from build123d import *

# Parameters (mm, degrees)
SKETCH1_W           = 60
SKETCH1_H           = 32
BOSS_EXTRUDE1_DEPTH = 1.2
BOSS_EXTRUDE2_DEPTH = 5.2
SKETCH3_W           = 10
SKETCH3_H           = 32
BOSS_EXTRUDE3_DEPTH = 1.2
SKETCH4_W           = 15
SKETCH4_H           = 10
BOSS_EXTRUDE4_DEPTH = 1.2
FILLET1_R           = 5
CUT_EXTRUDE1_REACH  = 59.861
SKETCH5_R           = 3.1


with BuildPart() as part:
    # Sketch1 → Boss-Extrude1 (new body)
    with BuildSketch(Plane(origin=(0, 0, 0), x_dir=(1, 0, 0), z_dir=(0, 1, 0))):
        Rectangle(SKETCH1_W, SKETCH1_H)
    extrude(amount=BOSS_EXTRUDE1_DEPTH)

    # Sketch2 → Boss-Extrude2 (add)
    with BuildSketch(Plane.XZ):
        Polygon((-30, -17.2), (31.2, -17.2), (31.2, 17.2), (-30, 17.2), (-30, 16), (30, 16), (30, -16), (-30, -16), align=None)
    extrude(amount=-BOSS_EXTRUDE2_DEPTH)

    # Sketch3 → Boss-Extrude3 (add)
    with BuildSketch(Plane.XZ):
        with Locations((-35, 0)):
            Rectangle(SKETCH3_W, SKETCH3_H)
    extrude(amount=-BOSS_EXTRUDE3_DEPTH)

    # Sketch4 → Boss-Extrude4 (add)
    with BuildSketch(Plane.XZ):
        with Locations((-47.5, 0)):
            Rectangle(SKETCH4_W, SKETCH4_H)
    extrude(amount=-BOSS_EXTRUDE4_DEPTH)

    # Fillet1
    fillet1_edges = [part.edges().sort_by_distance(p)[0] for p in [
        (-55, 0.6, 5),
        (-55, 0.6, -5),
    ]]
    fillet(fillet1_edges, radius=FILLET1_R - 0.0001)  # a hair under: the kernel refuses the full size

    # Sketch5 → Cut-Extrude1 (cut, up to next)
    with BuildSketch(Plane.XZ, mode=Mode.PRIVATE) as cut_extrude1_sk1:
        with Locations(Location((-50, 0, 0), (0, 0, 270))):
            Circle(SKETCH5_R)
    cut_extrude1_tool1 = extrude(cut_extrude1_sk1.sketch, amount=-CUT_EXTRUDE1_REACH, mode=Mode.PRIVATE) & part.part
    add(cut_extrude1_tool1.solids().sort_by_distance((-50, 0, 0))[0], mode=Mode.SUBTRACT)


solid = part.part
Input: part model. Units: mm. Frame: model coordinates. A direction names the side the tool comes from. Give positions to 0.01 mm unless a question says otherwise; leave off trailing zeros. Loops run counter-clockwise (first coordinate to the right, second up) from the corner with the lowest first, then second, coordinate; pieces in that order, holes last. Notation, with made-up numbers: (22.25, 22.25) -> (74.25, 22.25) arc R6 ccw to (74.25, 26.25) -> close; hole circle Ø9 at (89, -36). An arc over 180 degrees is marked (long way). Answer as a JSON object with one key per item and string values. Group by question number.
Item 1: Pin query (flat end, axial travel): P1, Ø1.3, axis at x = -46, y = 0.5, coming from the +Z side; P2, Ø1, axis at x = -45, y = 0.5, coming from the -Z side; P3, Ø1, axis at x = -36.5, y = 0.5, coming from the +Z side. Return the tip coordinate at first contact, or that it passes through.
Item 2: Cut plane C-C, the plane z = 15. Return the cut outline in (x, y), and give its area (3 significant figures).
Item 3: Cut plane A-A, the plane y = 4. Return the cut outline in (x, z), and give its area (3 significant figures).
Item 4: Line query: probe 1 along X at (y, z) = (0.7, 0); probe 2 along Z at (x, y) = (7.5, 2.3); probe 3 along Y at (x, z) = (9, -14.5). Output: solid intervals per line, ascending.
Item 5: Cut plane D-D, the plane z = 4. Return the cut outline in (x, y), and give its area (3 significant figures).
Item 6: Reachability of faces 1 (the flat face through (0, 3, 16)), 2 (the cylindrical face through (-46.926, 0.592, 0.404)) from +Z, -Z, +X, -X, +Y, -Y: full face, straight path, thin tool, end or side. Return the list, or none.
Item 7: Cut plane B-B, the plane x = -12. Return the cut outline in (y, z).
Checks:
{
 "1": {"P1": "stops at z = 5", "P2": "stops at z = -5", "P3": "stops at z = 16"},
 "2": {"outline": "(-40, 0) -> (31.2, 0) -> (31.2, 5.2) -> (30, 5.2) -> (30, 1.2) -> (-40, 1.2) -> close", "area": "90.2 mm²"},
 "3": {"outline": "(-30, -17.2) -> (31.2, -17.2) -> (31.2, 17.2) -> (-30, 17.2) -> (-30, 16) -> (30, 16) -> (30, -16) -> (-30, -16) -> close", "area": "185 mm²"},
 "4": {"probe 1": "x = -55 to -53.1, -46.9 to 31.2", "probe 2": "z = -17.2 to -16, 16 to 17.2", "probe 3": "y = 0 to 1.2"},
 "5": {"outline": "(-53, 0) -> (31.2, 0) -> (31.2, 5.2) -> (30, 5.2) -> (30, 1.2) -> (-53, 1.2) -> close", "area": "106 mm²"},
 "6": {"face 1": "-X, +Y", "face 2": "+Y, -Y"},
 "7": {"outline": "(0, -17.2) -> (5.2, -17.2) -> (5.2, -16) -> (1.2, -16) -> (1.2, 16) -> (5.2, 16) -> (5.2, 17.2) -> (0, 17.2) -> close"}
}
